Autodesk Fusion 360 part; units mm, degrees
sketch "Plate" plane through (0, 0, 0) normal (0, 1, 0) x (1, 0, 0) in component "Plate"
  line L0 (0, 0) -> (-22.8, 0)
  line L1 (-22.8, 0) -> (-22.8, 21.5)
  line L2 (-22.8, 21.5) -> (0, 38.25)
  line L3 (0, -20) -> (0, -2.5)
  line L4 (2.5, 0) -> (20, 0)
  line L5 (22.8, 21.5) -> (0, 38.25)
  line L6 (22.8, 0) -> (22.8, 21.5)
  line L7 (0, 0) -> (22.8, 0)
  point P0 (0, 38.25)
  dimension "d2" = 22.8
  dimension "d41" = 21.5
  dimension "d42" = 38.25
  dimension "d83" = 0
  dimension "d84" = 0
  dimension "d85" = 0
  dimension "d86" = 0
extrude "Extrude1" add sketch "Plate" along normal blind 5 makes body 1 in component "Plate"
fillet "Fillet3" radius 5 1 edges at (0, 2.5, -38.25) on bodies 1 in component "Plate"
fillet "Fillet4" radius 5 1 edges at (-22.8, 2.5, -21.5) on bodies 1 in component "Plate"
fillet "Fillet5" radius 5 1 edges at (22.8, 2.5, -21.5) on bodies 1 in component "Plate"
hole "Hole1" at (0, 5, -28.25) direction (0, -1, 0) diameter 8.5 end through all bodies 1 1 in component "Plate"
mirror "Mirror1" about plane through (0, 0, 0) normal (0, 0, 1) of bodies 1 makes body 2 in component "Plate"
combine "Combine1" operation add target body 1 tool bodies 2 in component "Plate"
hole "Hole1'" at (0, 5, 0) direction (0, -1, 0) diameter 10 end through all bodies 1 1 in component "Plate"
component "Plate" placed x (1, 0, 0) y (0, 1, 0) z (0, 0, 1) at (0, 0, 0)
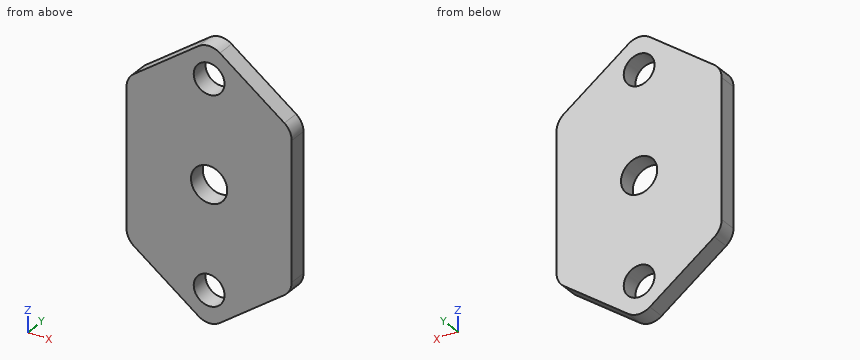
Here's how the part is built. I have some questions about the finished solid (model axes, mm). Give positions to 0.01 mm unless a question says otherwise; leave off trailing zeros. Order: outer loops, then holes, each group sorted by start corner. A loop starts at its lowest first (then second) coordinate and runs counter-clockwise, first axis right, second up. Notation, with made-up numbers: (62, 52.25) - (103, 52.25) arc R24 cw to (103, 69.25) - close; hole circle Ø5 at (53.25, 62). An arc over 180 degrees is marked (long way). Answer as a JSON object with one key per item and string values. Group by question number.
Item 1: For P1, Ø7, axis at x = 0, z = -28.25, coming from the -Y side; P2, Ø1, axis at x = -17.5, y = 4.5, coming from the +Z side, each with a flat end and sliding along its axis, tell me the tip position at first contact or that it passes through.
Item 2: If we section it at A-A on z = 0: Please give me the cut outline in (x, y).
Item 3: Please list where these lines run through material, in increasing order: probe 1 along Z at (x, y) = (0, 3.85); probe 2 along X at (y, z) = (1.1, 0); probe 3 along Z at (x, y) = (3, 4.55).
Item 4: If we section it at C-C on x = -1: Please give me the cut outline in (y, z), and give its area (3 significant figures).
Item 5: If we section it at B-B on y = 2.5: Please give me the cut outline in (x, z).
Item 6: If we section it at D-D on z = -31: Please give me the cut outline in (x, y).
Result set:
{
 "1": {"P1": "through", "P2": "z = 25.76"},
 "2": {"outline": "(-22.8, 0) - (-5, 0) - (-5, 5) - (-22.8, 5) - close; (5, 0) - (22.8, 0) - (22.8, 5) - (5, 5) - close"},
 "3": {"probe 1": "-37.05 to -32.5, -24 to -5, 5 to 24, 32.5 to 37.05", "probe 2": "-22.8 to -5, 5 to 22.8", "probe 3": "-36.05 to -31.26, -25.24 to -4, 4 to 25.24, 31.26 to 36.05"},
 "4": {"outline": "(0, -36.94) - (5, -36.94) - (5, -32.38) - (0, -32.38) - close; (0, -24.12) - (5, -24.12) - (5, -4.9) - (0, -4.9) - close; (0, 4.9) - (5, 4.9) - (5, 24.12) - (0, 24.12) - close; (0, 32.38) - (5, 32.38) - (5, 36.94) - (0, 36.94) - close", "area": "238 mm²"},
 "5": {"outline": "(-22.8, -18.97) arc R5 ccw to (-20.76, -23) - (-2.96, -36.08) arc R5 ccw to (2.96, -36.08) - (20.76, -23) arc R5 ccw to (22.8, -18.97) - (22.8, 18.97) arc R5 ccw to (20.76, 23) - (2.96, 36.08) arc R5 ccw to (-2.96, 36.08) - (-20.76, 23) arc R5 ccw to (-22.8, 18.97) - close; hole circle Ø10 at (0, 0); hole circle Ø8.5 at (0, -28.25); hole circle Ø8.5 at (0, 28.25)"},
 "6": {"outline": "(-9.87, 0) - (-3.24, 0) - (-3.24, 5) - (-9.87, 5) - close; (3.24, 0) - (9.87, 0) - (9.87, 5) - (3.24, 5) - close"}
}
